Here's how the part is built. I have some questions about the finished solid (model axes, mm). A direction names the side the tool comes from. Round coordinates to 2 decimals unless told otherwise and drop trailing zeros. Write each loop counter-clockwise with the first axis right and the second up, starting at its lowest first coordinate (ties: lowest second). Pieces come first, ordered by that corner, then holes. Notation, with made-up numbers: (-14.75, 46) -> (11.25, 46) arc R27 cw to (11.25, 65) -> close; hole circle Ø5 at (2.25, -35). An arc over 180 degrees is marked (long way). Answer in a Markdown table with one row per item.
from build123d import *

# Parameters (mm, degrees)
F0_W            = 210
F0_H            = 225
F1_DEPTH        = 25
F3_DEPTH        = 95
F4_R            = 37.5
F5_DEPTH        = 10
F5_DEPTH_BACK   = 125
F6_R            = 40
F7_DEPTH        = 10
F7_DEPTH_BACK   = 127
F8_W            = 60
F8_H            = 60
F9_DEPTH        = 10
F10_R           = 10
F12_DEPTH       = 20
F14_D           = 15
F14_CBORE_D     = 30
F14_CBORE_DEPTH = 10
F15_R           = 10
F16_R           = 19.5
F17_DEPTH       = 235.001
F18_R           = 19.5
F19_DEPTH       = 220.001
F20_SIZE        = 2
F21_R           = 10


with BuildPart() as f1:
    # F0 (on Top) → F1 (new body)
    with BuildSketch(Plane.XY):
        Rectangle(F0_W, F0_H)
    extrude(amount=F1_DEPTH)

    # F2 (on face) → F3 (join)
    with BuildSketch(Plane.XY.offset(25)):
        with BuildLine():
            ThreePointArc((25, 63.5), (-3.1177490061, -4.3822509939), (-71, -32.5))
            Line((-71, -32.5), (-71, -112.5))
            Line((-71, -112.5), (-56, -112.5))
            Line((-56, -112.5), (-56, -46.4818166789))
            ThreePointArc((-56, -46.4818166789), (7.4888527117, -14.9888527117), (38.9818166789, 48.5))
            Line((38.9818166789, 48.5), (105, 48.5))
            Line((105, 48.5), (105, 63.5))
            Line((105, 63.5), (25, 63.5))
        make_face()
    extrude(amount=F3_DEPTH)

    # F4 (on face) → F5 (join, two sides)
    with BuildSketch(Plane.XZ.offset(112.5)) as f5_sk:
        with Locations((-63.5, 120)):
            Circle(F4_R)
        with BuildLine():
            ThreePointArc((-56, 83.2576538583), (-63.5, 82.5), (-71, 83.2576538583))
            Line((-71, 83.2576538583), (-71, 25))
            Line((-71, 25), (-105, 25))
            Line((-105, 25), (-105, 0))
            Line((-105, 0), (105, 0))
            Line((105, 0), (105, 25))
            Line((105, 25), (-56, 25))
            Line((-56, 25), (-56, 83.2576538583))
        make_face()
    extrude(amount=F5_DEPTH)
    extrude(f5_sk.sketch, amount=-F5_DEPTH_BACK)

    # F6 (on face) → F7 (join, two sides)
    with BuildSketch(Plane.YZ.offset(105)) as f7_sk:
        with Locations((56, 120)):
            Circle(F6_R)
        with BuildLine():
            ThreePointArc((63.5, 80.7094158862), (86.8220700148, 94.504902432), (96, 120))
            ThreePointArc((96, 120), (30.504902432, 150.8220700148), (48.5, 80.7094158862))
            Line((48.5, 80.7094158862), (48.5, 120))
            Line((48.5, 120), (63.5, 120))
            Line((63.5, 120), (63.5, 80.7094158862))
        make_face()
    extrude(amount=F7_DEPTH)
    extrude(f7_sk.sketch, amount=-F7_DEPTH_BACK)

    # F8 (on face) → F9 (join)
    with BuildSketch(Plane.XY.offset(25)):
        with Locations((75, -92.5)):
            Rectangle(F8_W, F8_H)
    extrude(amount=F9_DEPTH)

    # F10
    f10_edges = [f1.edges().sort_by_distance(p)[0] for p in [
        (45, -62.5, 30),
    ]]
    fillet(f10_edges, radius=F10_R)

    # F11 (on face) → F12 (cut)
    with BuildSketch(Plane.XY.offset(25)):
        with BuildLine():
            ThreePointArc((46.5755076536, 39.5), (13.8528137424, -21.3528137424), (-47, -54.0755076536))
            Line((-47, -54.0755076536), (-47, -113.5))
            Line((-47, -113.5), (36, -113.5))
            Line((36, -113.5), (36, -72.5))
            ThreePointArc((36, -72.5), (41.5649711575, -59.0649711575), (55, -53.5))
            Line((55, -53.5), (96, -53.5))
            Line((96, -53.5), (96, 39.5))
            Line((96, 39.5), (46.5755076536, 39.5))
        make_face()
    extrude(amount=-F12_DEPTH, mode=Mode.SUBTRACT)

    # F14 (through all)
    with Locations(Plane.XY.offset(35)):
        with Locations((75, -92.5)):
            CounterBoreHole(F14_D / 2, F14_CBORE_D / 2, F14_CBORE_DEPTH)

    # F15
    f15_edges = [f1.edges().sort_by_distance(p)[0] for p in [
        (-47, -54.075508, 15),
        (46.575508, 39.5, 15),
        (-47, -113.5, 15),
        (96, 39.5, 15),
        (96, -53.5, 15),
        (36, -113.5, 15),
    ]]
    fillet(f15_edges, radius=F15_R)

    # F16 (on face) → F17 (cut, through all)
    with BuildSketch(Plane.XZ.offset(122.5)):
        with Locations((-63.5, 120)):
            Circle(F16_R)
    extrude(amount=-F17_DEPTH, mode=Mode.SUBTRACT)

    # F18 (on face) → F19 (cut, through all)
    with BuildSketch(Plane.YZ.offset(115)):
        with Locations((56, 120)):
            Circle(F18_R)
    extrude(amount=-F19_DEPTH, mode=Mode.SUBTRACT)

    # F20
    f20_edges = [f1.edges().sort_by_distance(p)[0] for p in [
        (115, 36.5, 120),
        (-83, -122.5, 120),
        (-22, 36.5, 120),
        (-83, 12.5, 120),
    ]]
    chamfer(f20_edges, length=F20_SIZE)

    # F21
    f21_edges = [f1.edges().sort_by_distance(p)[0] for p in [
        (105, 112.5, 12.5),
        (105, -122.5, 17.5),
        (-105, 112.5, 12.5),
        (-105, -122.5, 12.5),
    ]]
    fillet(f21_edges, radius=F21_R)


solid = f1.part
1) We'd pull the mould along X, two halves only. Please class faces 5 (the face through (102.15, 109.49, 12.68)), 6 (the face through (-18, -122.5, 20)), 7 (the face through (47.85, -65.51, 30.07)), 8 (the face through (49, -56, 25)): +X half, -X half, draft (parallel to the pull), parting line (faces both ways), or undercut.
Response:
| item | result |
|---|---|
| face 5 | +X half |
| face 6 | draft |
| face 7 | undercut |
| face 8 | undercut |
2) I need wall thicknesses on line 1 (Y direction, x = 75, z = 7); line 2 (Y direction, x = 75, z = 28.5); line 3 (X direction, y = -92, z = 27). Which ranges of each line are inside material? Lowest first, please. Write a range as [from, to].
Response:
| item | result |
|---|---|
| line 1 | y = [-122.5, -100], [-85, -53.5], [39.5, 112.5] |
| line 2 | y = [-122.5, -107.5], [-77.5, -62.5], [48.5, 63.5] |
| line 3 | x = [-71, -56], [45, 60.01], [89.99, 105] |
3) I want a section at A-A, the plane y = -92.5. List the corners of the cut face in (x, z) for me, and give its area (3 significant figures).
Response:
| item | result |
|---|---|
| outline | (-105, 0) -> (67.5, 0) -> (67.5, 25) -> (60, 25) -> (60, 35) -> (45, 35) -> (45, 25) -> (36, 25) -> (36, 5) -> (-47, 5) -> (-47, 25) -> (-56, 25) -> (-56, 83.26) arc R37.5 ccw (long way) to (-71, 83.26) -> (-71, 25) -> (-105, 25) -> close; (82.5, 0) -> (105, 0) -> (105, 35) -> (90, 35) -> (90, 25) -> (82.5, 25) -> close; hole circle Ø39 at (-63.5, 120) |
| area | 7,600 mm^2 |
4) I want a section at C-C, the plane x = 75. List the corners of the cut face in (y, z) for me.
Response:
| item | result |
|---|---|
| outline | (-122.5, 0) -> (-100, 0) -> (-100, 25) -> (-107.5, 25) -> (-107.5, 35) -> (-122.5, 35) -> close; (-85, 0) -> (112.5, 0) -> (112.5, 25) -> (63.5, 25) -> (63.5, 80.71) arc R40 ccw (long way) to (48.5, 80.71) -> (48.5, 25) -> (39.5, 25) -> (39.5, 5) -> (-53.5, 5) -> (-53.5, 25) -> (-62.5, 25) -> (-62.5, 35) -> (-77.5, 35) -> (-77.5, 25) -> (-85, 25) -> close; hole circle Ø39 at (56, 120) |
5) I want a section at B-B, the plane z = 31. List the corners of the cut face in (x, y) for me.
Response:
| item | result |
|---|---|
| outline | (-71, -122.5) -> (-56, -122.5) -> (-56, -46.48) arc R111 ccw to (38.98, 48.5) -> (105, 48.5) -> (105, 63.5) -> (25, 63.5) arc R96 cw to (-56, -31.32) -> (-56, 12.5) -> (-71, 12.5) -> close; (45, -122.5) -> (95, -122.5) arc R10 ccw to (105, -112.5) -> (105, -62.5) -> (55, -62.5) arc R10 ccw to (45, -72.5) -> close; hole circle Ø30 at (75, -92.5) |
6) Which directions (+Z, -Z, +X, -X, +Y, -Y) give clear straight access to the entire face, cutting with the end or side of a thin tool? Please do faces 1 (the face through (71.748, -107.143, 30.07)), 2 (the face through (105, -6, 16)), 3 (the face through (48.472, 37.497, 14.86)), 4 (the face through (6.77, -15.7, 71.84)).
Response:
| item | result |
|---|---|
| face 1 | +Z |
| face 2 | -Z, +X, +Y, -Y |
| face 3 | none |
| face 4 | +X, -Y |
7) For pin 1 (17.5 mm diameter, centred on y = -76, z = 54.5, fed in from +X); pin 2 (4 mm diameter, centred on y = -34, z = 107.5, fed in from -X); pin 3 (3 mm diameter, centred on x = 37.5, y = -29.5, fed in from +Z), each with a flat end and sliding along its axis, tell me the tip position at first contact or that it passes through.
Response:
| item | result |
|---|---|
| pin 1 | stops at x = -56 |
| pin 2 | stops at x = -99.5 |
| pin 3 | stops at z = 5 |
8) I want a section at D-D, the plane x = -63.5. List the corners of the cut face in (y, z) for me.
Response:
| item | result |
|---|---|
| outline | (-122.5, 0) -> (112.5, 0) -> (112.5, 25) -> (12.5, 25) -> (12.5, 98.5) -> (10.5, 100.5) -> (-120.5, 100.5) -> (-122.5, 98.5) -> close; (-122.5, 141.5) -> (-120.5, 139.5) -> (10.5, 139.5) -> (12.5, 141.5) -> (12.5, 157.5) -> (-122.5, 157.5) -> close |
